Autodesk Inventor part; units mm, degrees
ref_plane "YZ Plane" through (0, 0, 0) normal (1, 0, 0) x (0, 1, 0)
ref_plane "XZ Plane" through (0, 0, 0) normal (0, 1, 0) x (-1, 0, 0)
ref_plane "XY Plane" through (0, 0, 0) normal (0, 0, 1) x (1, 0, 0)
sketch "Sketch1" plane through (0, 0, 0) normal (0, 1, 0) x (-1, 0, 0)
  line L0 (-126.3701, 48.161) -> (-51.2671, 4.8003) construction
  line L1 (-51.2671, 4.8003) -> (-126.3701, -38.5605) construction
  line L2 (-126.3701, -38.5605) -> (-126.3701, 48.161) construction
  line L3 (110.9585, 0) -> (-59.5814, 0) construction
  line L4 (83.2089, 69.641) -> (63.2089, 35)
  line L5 (63.2089, 35) -> (-58.0347, 105)
  line L6 (-58.0347, 105) -> (-68.0347, 87.6795)
  line L7 (-68.0347, 87.6795) -> (-50.7142, 77.6795)
  line L8 (-33.3937, 67.6795) -> (40.2185, 25.1795)
  line L9 (83.2089, -69.641) -> (63.2089, -35)
  line L10 (63.2089, -35) -> (-58.0347, -105)
  line L11 (-58.0347, -105) -> (-68.0347, -87.6795)
  line L12 (-68.0347, -87.6795) -> (-50.7142, -77.6795)
  line L13 (-33.3937, -67.6795) -> (40.2185, -25.1795)
  arc A0 (83.2089, -69.641) -> (83.2089, 69.641) centre (55.3678, 0) ccw
  line L14 (-50.7142, 77.6795) -> (-50.7142, -77.6795)
  line L15 (-33.3937, 67.6795) -> (-33.3937, -67.6795)
  line L16 (40.2185, 25.1795) -> (40.2185, -25.1795)
  dimension "d3" = 40
  dimension "d4" = 140
  dimension "d5" = 20
  dimension "d7" = 20
  dimension "d19" = 70
  dimension "d20" = 75
  dimension "d21" = 20
  dimension "d22" = 85
extrude "Extrusion1" add sketch "Sketch1" along normal blind 40
sketch "Sketch2" plane through (-63.2089, 0, 35) normal (0.866, 0, 0.5) x (0.5, 0, -0.866)
  circle A0 centre (-20, 20) radius 3.4
  line L0 (-40, 40) -> (0, 40)
  line L1 (-40, 0) -> (-40, 40)
  point P0 (61.9153, 0)
  point P1 (-20, 40)
  point P2 (-40, 20)
  dimension "d10" = 6.8
extrude "Extrusion2" add sketch "Sketch2" along normal blind 10
sketch "Sketch3" plane through (-83.2089, 0, -69.641) normal (0.866, 0, -0.5) x (-0.5, 0, -0.866)
  circle A0 centre (-20, 20) radius 3.4
  line L0 (-40, 40) -> (0, 40)
  line L1 (0, 0) -> (0, 40)
  point P0 (-101.9153, 0)
  point P1 (-20, 40)
  point P2 (0, 20)
  dimension "d13" = 6.8
extrude "Extrusion3" add sketch "Sketch3" along normal blind 10
sketch "Sketch4" plane through (0, 40, 0) normal (0, 1, 0) x (1, 0, 0)
  line L0 (-105.2185, -20) -> (-65.2185, -20)
  line L1 (-65.2185, -20) -> (-65.2185, 20)
  line L2 (-65.2185, 20) -> (-105.2185, 20)
  line L3 (-105.2185, 20) -> (-105.2185, -20)
  line L4 (-40.2185, -25.1795) -> (-40.2185, 25.1795)
  point P0 (0, 0)
  point P1 (-105.2185, 0)
  dimension "d16" = 40
  dimension "d17" = 40
  dimension "d23" = 25
extrude "Extrusion4" cut sketch "Sketch4" against normal blind 40
fillet "Fillet1" radius 10 2 edges at (-40.2185, 20, -25.1795) (-40.2185, 20, 25.1795)
fillet "Fillet2" radius 13 2 edges at (33.3937, 20, 67.6795) (33.3937, 20, -67.6795)
fillet "Fillet3" radius 15 2 edges at (50.7142, 20, 77.6795) (50.7142, 20, -77.6795)
sketch "Sketch5" plane through (68.0347, 0, 87.6795) normal (0.5, 0, -0.866) x (-0.866, 0, -0.5)
  point P0 (102.7595, 0)
  point P1 (5.815, 19.918)
hole "Hole1" at (62.9988, 19.918, 84.772) direction (-0.5, 0, 0.866) diameter 4 end through all counterbore diameter 5 counterbore depth 2
sketch "Sketch6" plane through (-35.2185, 0, 28.0662) normal (0.5, 0, -0.866) x (-0.866, 0, -0.5)
  point P0 (-16.467, 0)
  point P1 (-7.7378, 18.9937)
hole "Hole2" at (-28.5174, 18.9937, 31.9351) direction (-0.5, 0, 0.866) diameter 4 end through all counterbore diameter 5 counterbore depth 2
fillet "Fillet8" radius 1 16 edges at (-10.6624, 0, 42.2437) (33.3937, 0, 0) (-10.6624, 0, -42.2437) (-40.2185, 0, 0) (63.1244, 0, -84.8446) (63.1244, 0, 84.8446) (50.7142, 0, 0) (-10.6624, 40, -42.2437) (33.3937, 40, 0) (-10.6624, 40, 42.2437) (-40.2185, 40, 0) (63.1244, 40, -84.8446) (63.1244, 40, 84.8446) (50.7142, 40, 0) (68.0347, 20, 87.6795) (68.0347, 20, -87.6795)
fillet "Fillet9" radius 1 2 edges at (-130.3678, 0, 0) (-130.3678, 40, 0)
sketch "Sketch8" plane through (50.7142, 1, 69.0192) normal (1, 0, 0) x (0, 0, -1)
  circle A0 centre (34.0192, 18) radius 7.5
  circle A1 centre (104.0192, 18) radius 7.5
  line L0 (97.0855, 0) -> (97.0855, 38)
  line L1 (0, 38) -> (138.0385, 38)
  circle A2 centre (69.0192, 18) radius 5
  point P0 (69.0192, -1)
  dimension "d56" = 15
  dimension "d57" = 15
  dimension "d58" = 20
  dimension "d59" = 35
  dimension "d60" = 35
  dimension "d82" = 10
sketch "Sketch9" plane through (-40.2185, 1, 19.406) normal (1, 0, 0) x (0, 0, -1)
  line L0 (0, 38) -> (38.812, 38)
  line L1 (19.406, 38) -> (19.406, 0) construction
  line L2 (38.812, 0) -> (0, 0)
  line L3 (0, 19) -> (38.812, 19) construction
  line L4 (0, 0) -> (0, 38)
  line L5 (38.812, 38) -> (38.812, 0)
  point P0 (19.406, -1)
  point P1 (3.906, 34.5)
  point P2 (34.906, 34.5)
  point P3 (3.906, 3.5)
  point P4 (34.906, 3.5)
  dimension "d64" = 19
  dimension "d67" = 15.5
  dimension "d68" = 15.5
  dimension "d69" = 15.5
  dimension "d70" = 15.5
  dimension "d71" = 15.5
  dimension "d72" = 15.5
  dimension "d73" = 15.5
  dimension "d74" = 15.5
hole "Hole4" at (-40.2185, 35.5, 15.5) at (-40.2185, 35.5, -15.5) at (-40.2185, 4.5, 15.5) at (-40.2185, 4.5, -15.5) direction (-1, 0, 0) diameter 4 depth 15 tip angle 118
extrude "Extrusion6" cut sketch "Sketch8" against normal blind 20
properties part number "Profil_Winkel_oben"
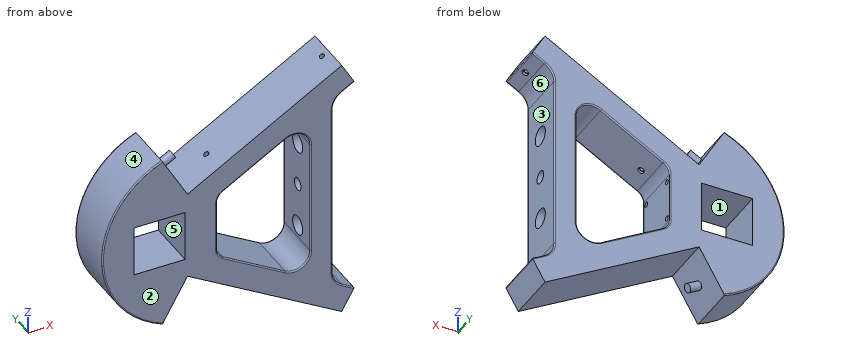
Build history of the part. All positions in model axes, mm. Face numbers are marked on the shaded views. A direction names the side the tool comes from. Round coordinates to 2 decimals unless told otherwise and drop trailing zeros. Order: outer loops, then holes, each group sorted by start corner. A loop starts at its lowest first (then second) coordinate and runs counter-clockwise, first axis right, second up. Notation, with made-up numbers: M 41.5,-16 L 60.5,-16 A16 ccw 60.5,12 Z; hole C 82,10 d1. An arc over 180 degrees is marked long. Use CSV: the item, a comma, the result in double quotes. Start each with the question number.
(1) Flat gauge pins, fed straight in: P1, Ø6, axis at x = -84.5, y = 24.5, coming from the -Z side; P2, Ø16, axis at y = 19, z = 0, coming from the +X side; P3, Ø4.5, axis at y = 4.5, z = 15.5, coming from the -X side. Where does each tip first touch, or does it go through?
(2) Drill centre lines: probe 1 along Y at (x, z) = (-47.75, 15.5); probe 2 along Z at (x, y) = (41, 18.5); probe 3 along X at (y, z) = (27.5, 8). Where is each one in solid material? Low to high.
(3) Cut at A-A on z = 0. List the corners of the cut face in (x, y), then the cut area to 3 significant figures.
(4) Mould opens along X. For the marked faces 4, 5 and 6 say: +X half, -X half, draft (parallel to the pull), parting line (faces both ways), or undercut.
(5) Tool access for the marked faces 1, 2 and 3: list every direction of +Z, -Z, +X, -X, +Y, -Y with a clear straight run to the whole face (end or side of a thin tool).
Findings:
1,P1,"stops at z = -69.64"
1,P2,"stops at x = 50.71"
1,P3,"stops at x = -129.19"
2,probe 1,"y = 0 to 2.5, 6.5 to 33.5, 37.5 to 40"
2,probe 2,"z = -95.17 to -42.48, -27.52 to -4.97, 4.97 to 27.52, 42.48 to 95.17"
2,probe 3,"x = -129.94 to -105.22, -65.22 to -40.22, 33.39 to 50.71"
3,outline,"M -130.37,1 A1 ccw -129.37,0 L -105.22,0 L -105.22,40 L -129.37,40 A1 ccw -130.37,39 Z; M -65.22,0 L -41.22,0 A1 ccw -40.22,1 L -40.22,39 A1 ccw -41.22,40 L -65.22,40 Z; M 33.39,1 A1 ccw 34.39,0 L 49.71,0 A1 ccw 50.71,1 L 50.71,14 L 33.39,14 Z; M 33.39,24 L 50.71,24 L 50.71,39 A1 ccw 49.71,40 L 34.39,40 A1 ccw 33.39,39 Z"
3,area,"2,520 mm^2"
4,face 4,"-X half"
4,face 5,"undercut"
4,face 6,"+X half"
5,face 1,"+Y, -Y"
5,face 2,"+Z, -Z, +X, -X, -Y"
5,face 3,"+X, +Y, -Y"
